Read the model definition and answer for the solid it produces. Units are mm, in the model's axes. Face numbers are marked on the shaded views. Round coordinates to 2 decimals unless told otherwise and drop trailing zeros. Order: outer loops, then holes, each group sorted by start corner. A loop starts at its lowest first (then second) coordinate and runs counter-clockwise, first axis right, second up. Notation, with made-up numbers: (47.25, 10) -> (106.25, 10) arc R20 ccw to (106.25, 44) -> close; hole circle Ø4 at (53.25, -28). An arc over 180 degrees is marked (long way). Use a Markdown table: item, result. Add a question column.
1. Section B-B, the plane z = 27 is taken. Give the vertices of the cut face in (x, y).
2. Given pin 1 (5.5 mm diameter, centred on x = -25.5, y = 24.5, fed in from -Z); pin 2 (2 mm diameter, centred on x = -43, z = 85, fed in from -Y); pin 3 (6 mm diameter, centred on y = 31.5, z = 52, fed in from +X), each flat-ended and moving along its own axis, determine where each tip first touches the part or whether it passes through.
3. The mould has two halves that part along X. Classify the marked faces 1, 2, 3 and 4: +X half, -X half, draft (parallel to the pull), parting line (faces both ways), or undercut.
4. Section A-A, the plane y = 25 is taken. Give the vertices of the cut face in (x, z), then the cut area to 3 significant figures.
5. Consider L1, parallel to Y at x = -25, z = 72; L2, parallel to X at y = 25, z = 64; L3, parallel to Y at x = -25, z = 87.25. Determine where each line is inside the solid, lowest interval first. Write a range as [from, to].
6. Section C-C, the plane x = -25 is taken. Give the vertices of the cut face in (y, z).
7. Section D-D, the plane x = -5 is taken. Give the vertices of the cut face in (y, z), then the cut area to 3 significant figures.
Autodesk Fusion 360 part; units mm, degrees
sketch "Sketch1" plane through (0, 0, 0) normal (0, 0, 1) x (1, 0, 0)
  line L0 (0, 0) -> (-50, 0)
  line L1 (-50, 0) -> (-50, 50)
  line L2 (-50, 50) -> (0, 50)
  line L3 (0, 50) -> (0, 0)
  dimension "d1" = 50
  dimension "d2" = 50
extrude "Extrude1" add sketch "Sketch1" along normal blind 100
ref_plane "WorkPlane1" through (-25, 25, 0) normal (0, 0, -1) x (-1, 0, 0)
sketch "Sketch2" plane through (-25, 25, 0) normal (0, 0, -1) x (1, 0, 0)
  circle A0 centre (0, 0) radius 12.5
  dimension "d6" = 25
extrude "Extrude2" cut sketch "Sketch2" against normal blind 50 draft -20
sketch "Sketch3" plane through (0, 0, 0) normal (0, 0, -1) x (1, 0, 0)
  circle A0 centre (-25, -25) radius 12.5
  line L0 (-50, -50) -> (0, -50)
  line L1 (0, -50) -> (0, 0)
  line L2 (0, 0) -> (-50, 0)
  line L3 (-50, 0) -> (-50, -50)
ref_plane "WorkPlane2" through (-25, 25, 0) normal (0, 0, -1) x (1, 0, 0)
sketch "Sketch4" plane through (0, 0, 0) normal (0, 0, -1) x (1, 0, 0)
  circle A0 centre (-25, -25) radius 3
  circle A1 centre (-25, -25) radius 4.75
  dimension "d10" = 6
  dimension "d11" = 9.5
extrude "Extrude3" cut sketch "Sketch4" against normal blind 100 contours A0
sketch "Sketch5" plane through (-25, 25, 0) normal (0, 0, -1) x (1, 0, 0)
  circle A0 centre (0, 0) radius 4.75
  dimension "d14" = 9.5
extrude "Extrude4" cut sketch "Sketch5" against normal blind 80
sketch "Sketch6" plane through (0, 0, 0) normal (0, 0, -1) x (1, 0, 0)
ref_plane "WorkPlane3" through (0, 25, 50) normal (1, 0, 0) x (0, 1, 0)
sketch "Sketch7" plane through (0, 25, 50) normal (1, 0, 0) x (0, 1, 0)
  line L0 (-25, -50) -> (-20, -50)
  line L1 (-20, -50) -> (-20, -37)
  line L2 (-20, -37) -> (-25, -37)
  line L3 (-25, -37) -> (-25, -50)
  line L4 (-25, -37) -> (-20, -37)
  line L5 (-20, -37) -> (-20, -23)
  line L6 (-20, -23) -> (-25, -23)
  line L7 (-25, -23) -> (-25, -37)
  circle A0 centre (-20, -23) radius 2.4
  circle A1 centre (-20, -37) radius 2.4
  dimension "d18" = 5
  dimension "d19" = 13
  dimension "d20" = 5
  dimension "d21" = 14
  dimension "d22" = 4.8
  dimension "d23" = 4.8
extrude "Extrude5" add sketch "Sketch7" along normal blind 2 contours L1 L2 L4 A1 | L1 L5 A1 | L2 L4 L5 A1 | L5 L6 A0 | L5 L6 A0
ref_plane "WorkPlane4" through (-25, 0, 50) normal (0, -1, 0) x (1, 0, 0)
sketch "Sketch8" plane through (-25, 0, 50) normal (0, -1, 0) x (1, 0, 0)
  line L0 (25, -50) -> (20, -50)
  line L1 (20, -50) -> (20, -37)
  line L2 (20, -37) -> (25, -37)
  line L3 (25, -37) -> (25, -50)
  line L4 (25, -37) -> (20, -37)
  line L5 (20, -37) -> (20, -23)
  line L6 (20, -23) -> (25, -23)
  line L7 (25, -23) -> (25, -37)
  circle A0 centre (20, -23) radius 2.4
  circle A1 centre (20, -37) radius 2.4
  dimension "d27" = 4.8
  dimension "d28" = 4.8
extrude "Extrude6" add sketch "Sketch8" along normal blind 2 contours L1 L5 A1 | L1 L2 L4 A1 | L2 L4 L5 A1 | L5 L6 A0 | L5 L6 A0
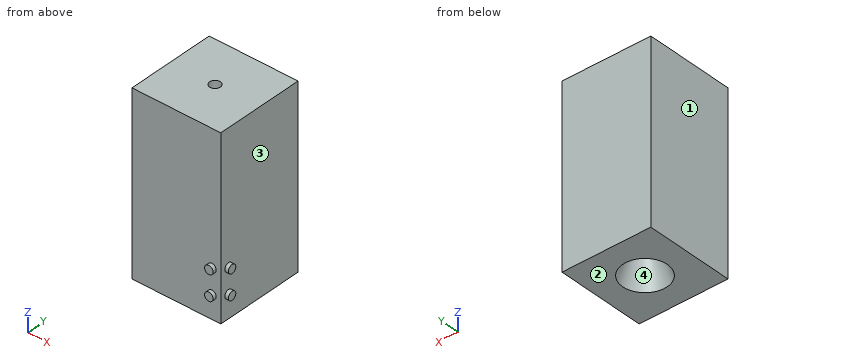
Verdict:
| question | item | result |
|---|---|---|
| 1 | outline | (-50, 0) -> (-7.4, 0) -> (-7.4, -2) -> (-2.6, -2) -> (-2.6, 0) -> (0, 0) -> (0, 2.6) -> (2, 2.6) -> (2, 7.4) -> (0, 7.4) -> (0, 50) -> (-50, 50) -> close; hole circle Ø9.5 at (-25, 25) |
| 2 | pin 1 | stops at z = 80 |
| 2 | pin 2 | stops at y = 0 |
| 2 | pin 3 | stops at x = 0 |
| 3 | face 1 | -X half |
| 3 | face 2 | draft |
| 3 | face 3 | +X half |
| 3 | face 4 | undercut |
| 4 | outline | (-50, 0) -> (-37.5, 0) -> (-29.75, 21.29) -> (-29.75, 47.39) -> (-30.7, 50) -> (-29.75, 50) -> (-29.75, 80) -> (-28, 80) -> (-28, 100) -> (-50, 100) -> close; (-22, 80) -> (-20.25, 80) -> (-20.25, 50) -> (-19.3, 50) -> (-20.25, 47.39) -> (-20.25, 21.29) -> (-12.5, 0) -> (0, 0) -> (0, 100) -> (-22, 100) -> close |
| 4 | area | 3,950 mm2 |
| 5 | L1 | y = [0, 20.25], [29.75, 50] |
| 5 | L2 | x = [-50, -29.75], [-20.25, 0] |
| 5 | L3 | y = [0, 22], [28, 50] |
| 6 | outline | (0, 0) -> (12.5, 0) -> (20.25, 21.29) -> (20.25, 47.39) -> (19.3, 50) -> (20.25, 50) -> (20.25, 80) -> (22, 80) -> (22, 100) -> (0, 100) -> close; (28, 80) -> (29.75, 80) -> (29.75, 50) -> (30.7, 50) -> (29.75, 47.39) -> (29.75, 21.29) -> (37.5, 0) -> (50, 0) -> (50, 100) -> (28, 100) -> close |
| 7 | outline | (-2, 10.6) -> (0, 10.6) -> (0, 0) -> (50, 0) -> (50, 100) -> (0, 100) -> (0, 29.4) -> (-2, 29.4) -> (-2, 24.6) -> (0, 24.6) -> (0, 15.4) -> (-2, 15.4) -> close |
| 7 | area | 5,020 mm2 |
